Autodesk Inventor part; units mm, degrees
ref_plane "YZ Plane" through (0, 0, 0) normal (1, 0, 0) x (0, 1, 0)
ref_plane "XZ Plane" through (0, 0, 0) normal (0, 1, 0) x (-1, 0, 0)
ref_plane "XY Plane" through (0, 0, 0) normal (0, 0, 1) x (1, 0, 0)
sketch "Sketch1" plane through (0, 0, 0) normal (0, 1, 0) x (-1, 0, 0)
  line L0 (-7.8, 14.985) -> (7.8, 14.985)
  line L1 (7.8, 14.985) -> (7.8, -14.985)
  line L2 (7.8, -14.985) -> (-7.8, -14.985)
  line L3 (-7.8, -14.985) -> (-7.8, 14.985)
  line L4 (-7.8, 14.985) -> (7.8, -14.985) construction
  line L5 (7.8, 14.985) -> (-7.8, -14.985) construction
  point P0 (0, 0)
  dimension "d0" = 15.6
  dimension "d1" = 29.97
extrude "Extrusion1" add sketch "Sketch1" along normal mid plane 0.8
sketch "Sketch2" plane through (0, 0.4, 0) normal (0, 1, 0) x (1, 0, 0)
  line L0 (-7.8, -14.985) -> (7.8, -14.985)
  line L1 (7.8, -14.985) -> (7.8, 14.985)
  line L2 (7.8, 14.985) -> (-7.8, 14.985)
  line L3 (-7.8, 14.985) -> (-7.8, -14.985)
  line L4 (7.8, 14.985) -> (-7.8, 14.985)
  line L5 (7.8, -14.985) -> (7.8, 14.985)
  line L6 (-7.8, 14.985) -> (7.8, 14.985)
  line L7 (7.8, 14.985) -> (7.8, -10.015)
  line L8 (7.8, -10.015) -> (-7.8, -10.015)
  line L9 (-7.8, -10.015) -> (-7.8, 14.985)
  point P0 (0, 0)
  dimension "d4" = 25
extrude "Extrusion2" add sketch "Sketch2" along normal blind 5.86 and the other way blind 2.75 contours L3 L2 L1 L8
properties part number "Module_CO2Sensor-T6713" material "ABS Plastic"
Input: part model. Units: mm. Frame: model coordinates. A direction names the side the tool comes from. Round coordinates to 2 decimals unless told otherwise and drop trailing zeros. Write each loop counter-clockwise with the first axis right and the second up, starting at its lowest first coordinate (ties: lowest second). Pieces come first, ordered by that corner, then holes. Notation, with made-up numbers: (-5, 19) -> (12, 19) arc R8 ccw to (12, 30) -> close; hole circle Ø6 at (33.25, 29.25). An arc over 180 degrees is marked (long way). Answer as CSV lines item,"result".
1. Section C-C (z = 12.5). Return the cut outline in (x, y), plus the area to 3 significant figures.
Geometry says:
outline,"(-7.8, -0.4) -> (7.8, -0.4) -> (7.8, 0.4) -> (-7.8, 0.4) -> close"
area,"12.5 mm^2"
2. Section B-B (y = -2). Return the cut outline in (x, z) (3 decimals).
Geometry says:
outline,"(-7.8, -14.985) -> (7.8, -14.985) -> (7.8, 10.015) -> (-7.8, 10.015) -> close"
3. Reachability of faces 1 (the flat face through (0, -2.35, -3)), 2 (the flat face through (0, -0.4, 13)), 3 (the flat face through (0, 0.4, 13)) from +Z, -Z, +X, -X, +Y, -Y: full face, straight path, thin tool, end or side. Return the list, or none.
Geometry says:
face 1,"+Z, -Z, +X, -X, -Y"
face 2,"+Z, +X, -X, -Y"
face 3,"+Z, +X, -X, +Y"
4. Section A-A (x = -4.25). Return the cut outline in (y, z) (3 decimals).
Geometry says:
outline,"(-2.35, -14.985) -> (6.26, -14.985) -> (6.26, 10.015) -> (0.4, 10.015) -> (0.4, 14.985) -> (-0.4, 14.985) -> (-0.4, 10.015) -> (-2.35, 10.015) -> close"
5. Contact query for flat-ended pins moving along their axis: P1, Ø1.8, axis at x = -3.5, y = 3.5, coming from the +Z side (3 decimals); P2, Ø1.5, axis at x = -2, z = 12.5, coming from the +Y side. Output: stop coordinate, or through.
Geometry says:
P1,"stops at z = 10.015"
P2,"stops at y = 0.4"
6. Ray query, L1, parallel to Z at x = 4.25, y = 3.5 (3 decimals); L2, parallel to Y at x = -6, z = 10.25. Return the intervals inside material, ascending. Write a range as [from, to].
Geometry says:
L1,"z = [-14.985, 10.015]"
L2,"y = [-0.4, 0.4]"
